The listing builds one solid part. Answer for the finished solid, in the listing's coordinates (mm). A direction names the side the tool comes from. Coordinates: 2 decimals unless noted, no trailing zeros. Order: outer loops, then holes, each group sorted by start corner. A loop starts at its lowest first (then second) coordinate and runs counter-clockwise, first axis right, second up. Notation, with made-up numbers: (22.25, 13.5) -> (26.25, 13.5) arc R28 cw to (26.25, 46.5) -> close; hole circle Ø5 at (84.5, -4). An arc over 180 degrees is marked (long way). Write each question's results on one line, items separated by ' | '. Start each with the question number.
(1) Determine the mould class of faces 1 (the face through (7.29, -14.02, 41.99)), 2 (the face through (-61.005, 274.722, -18.583)), 3 (the face through (-61.08, 275.06, 18.75)) for opening direction Z: +Z half, -Z half, draft (parallel to the pull), parting line (faces both ways), or undercut.
(2) A tool of negligible diameter and unlimited length cuts with its end or side. For faces 4 (the face through (-4.336, -19.524, -45.465)), 5 (the face through (15, 6, -43)), 6 (the face through (-4.336, -19.524, 45.465)), from which of +Z, -Z, +X, -X, +Y, -Y can it reach the whole face along a straight path? Write none if from no direction.
(3) Given pin 1 (6 mm diameter, centred on x = -22, z = 13.5, fed in from +Y); pin 2 (4 mm diameter, centred on y = 29, z = 1, fed in from -X), each flat-ended and moving along its own axis, determine where each tip first touches the part or whether it passes through.
(4) The part is cut by section C-C, the plane z = -57. Give the vertices of the cut face in (x, y).
(5) The part is cut by section A-A, the plane x = 71.5. Count the separate pieces of the cut face and the enclosed holes in it, then the cut area to 3 significant figures.
(6) Straight lines are drawn through the part: L1, parallel to Y at x = 0, z = 1; L2, parallel to X at y = 229.5, z = -2.5; L3, parallel to Y at x = 3, z = 26.5. For each, find the intervals that lie inside material, in ascending order.
```python
from build123d import *

# Parameters (mm, degrees)
SKETCH1_R            = 15
BOSS_EXTRUDE1_DEPTH  = 38
SKETCH2_R            = 15
BOSS_EXTRUDE2_DEPTH  = 3
BOSS_EXTRUDE2_DRAFT  = -15
SKETCH3_R            = 15.803847577
BOSS_EXTRUDE3_DEPTH  = 2
SKETCH4_R            = 20
BOSS_EXTRUDE4_DEPTH  = 5
SKETCH5_R            = 5
BOSS_EXTRUDE5_DEPTH  = 40
BOSS_EXTRUDE14_DEPTH = 10


with BuildPart() as part:
    # Sketch1 → Boss-Extrude1 (new body)
    with BuildSketch(Plane.XY):
        Circle(SKETCH1_R)
    extrude(amount=BOSS_EXTRUDE1_DEPTH)


with BuildPart() as boss_extrude2_tool:
    # Sketch2 → Boss-Extrude2 (with draft: the straight prism first)
    with BuildSketch(Plane.XY.offset(38)):
        Circle(SKETCH2_R)
    extrude(amount=BOSS_EXTRUDE2_DEPTH)
    # Boss-Extrude2: the draft: its side faces are tilted about the plane it starts from
    boss_extrude2_sides = [boss_extrude2_tool.faces().sort_by_distance(p)[0] for p in [
        (-15, 0, 39.5),
    ]]
    draft(boss_extrude2_sides, Plane.XY.offset(38), BOSS_EXTRUDE2_DRAFT)


with BuildPart() as part_1:
    add(part.part)

    # Boss-Extrude2: add boss_extrude2_tool
    add(boss_extrude2_tool.part)

    # Sketch3 → Boss-Extrude3 (add)
    with BuildSketch(Plane.XY.offset(41)):
        Circle(SKETCH3_R)
    extrude(amount=BOSS_EXTRUDE3_DEPTH)

    # Sketch4 → Boss-Extrude4 (add)
    with BuildSketch(Plane.XY.offset(43)):
        Circle(SKETCH4_R)
    extrude(amount=BOSS_EXTRUDE4_DEPTH)

    # Sketch5 → Boss-Extrude5 (add)
    with BuildSketch(Plane.XY.offset(48)):
        Circle(SKETCH5_R)
    extrude(amount=BOSS_EXTRUDE5_DEPTH)

    # Mirror1: part across plane


with BuildPart() as part_2:
    add(part_1.part)
    add(part_1.part.mirror(Plane.XY))



with BuildPart() as body_2:
    # Sketch6 → Revolve1 (revolve)
    with BuildSketch(Plane(origin=(0, 0, 0), x_dir=(0, 0, -1), z_dir=(1, 0, 0)), mode=Mode.PRIVATE) as revolve1_sk:
        Polygon((-30, 305.2), (30, 305.2), (18, 280.2), (-18, 280.2), align=None)
    revolve(revolve1_sk.sketch.rotate(Axis((0, 0, 38), (0, 0, -1)), 90), axis=Axis((0, 0, 38), (0, 0, -1)))


with BuildPart() as part_3:
    add(part_2.part)

    add(body_2.part)  # Boss-Extrude14 merges body 2
    # Sketch7 → Boss-Extrude14 (add, symmetric)
    with BuildSketch(Plane.XY):
        with BuildLine():
            ThreePointArc((-7.320383178, 13.09244019), (-25.622638941, 148.911014187), (15, 279.798213004))
            ThreePointArc((15, 279.798213004), (70.845559028, 271.0958258), (123.808589933, 251.363229329))
            ThreePointArc((123.808589933, 251.363229329), (36.300695478, 146.53460966), (7.320383178, 13.09244019))
            ThreePointArc((7.320383178, 13.09244019), (0, 15), (-7.320383178, 13.09244019))
        make_face()
        with BuildLine():
            ThreePointArc((13.09244019, 7.320383178), (148.911014187, 25.622638941), (279.798213004, -15))
            ThreePointArc((279.798213004, -15), (271.0958258, -70.845559028), (251.363229329, -123.808589933))
            ThreePointArc((251.363229329, -123.808589933), (146.53460966, -36.300695478), (13.09244019, -7.320383178))
            ThreePointArc((13.09244019, -7.320383178), (15, 0), (13.09244019, 7.320383178))
        make_face()
        with BuildLine():
            ThreePointArc((7.320383178, -13.09244019), (25.622638941, -148.911014187), (-15, -279.798213004))
            ThreePointArc((-15, -279.798213004), (-70.845559028, -271.0958258), (-123.808589933, -251.363229329))
            ThreePointArc((-123.808589933, -251.363229329), (-36.300695478, -146.53460966), (-7.320383178, -13.09244019))
            ThreePointArc((-7.320383178, -13.09244019), (0, -15), (7.320383178, -13.09244019))
        make_face()
        with BuildLine():
            ThreePointArc((-13.09244019, -7.320383178), (-148.911014187, -25.622638941), (-279.798213004, 15))
            ThreePointArc((-279.798213004, 15), (-271.0958258, 70.845559028), (-251.363229329, 123.808589933))
            ThreePointArc((-251.363229329, 123.808589933), (-146.53460966, 36.300695478), (-13.09244019, 7.320383178))
            ThreePointArc((-13.09244019, 7.320383178), (-15, 0), (-13.09244019, -7.320383178))
        make_face()
    extrude(amount=BOSS_EXTRUDE14_DEPTH, both=True)

    # Sketch8 → Revolve2 (revolve)
    with BuildSketch(Plane(origin=(0, 0, 0), x_dir=(1, 0, 0), z_dir=(0, 1, 0))):
        with BuildLine():
            Line((305.2, 30), (305.2, -30))
            ThreePointArc((305.2, -30), (335.2, 0), (305.2, 30))
        make_face()
    revolve(axis=Axis((0, 0, 38), (0, 0, -1)))


solid = part_3.part
```
Established:
1) face 1: undercut | face 2: -Z half | face 3: +Z half
2) face 4: -Z | face 5: none | face 6: +Z
3) pin 1: stops at y = 332.59 | pin 2: stops at x = -334.1
4) outline: circle Ø10 at (0, 0)
5) separate pieces: 3 | enclosed holes: 0 | area: 7,450 mm^2
6) L1: y = -335.18 to -280.2, -249.96 to 249.96, 280.2 to 335.18 | L2: x = -244.17 to -160.75, -8.14 to 97.54, 160.75 to 244.17 | L3: y = -319.25 to -297.89, -14.7 to 14.7, 297.89 to 319.25
